from build123d import *

# Parameters (mm, degrees)
F0_R     = 9.95
F1_DEPTH = 3


with BuildPart() as f1:
    # F0 (on Top) → F1 (new body)
    with BuildSketch(Plane.XY):
        with BuildLine():
            ThreePointArc((14.825089, -2.284017), (14.743027, 2.764626), (12.990381, 7.5))
            ThreePointArc((12.990381, 7.5), (9.76575, 11.385523), (5.434528, 13.980912))
            ThreePointArc((5.434528, 13.980912), (0, 45.080944), (-5.434528, 13.980912))
            ThreePointArc((-5.434528, 13.980912), (-9.76575, 11.385523), (-12.990381, 7.5))
            ThreePointArc((-12.990381, 7.5), (-14.743027, 2.764626), (-14.825089, -2.284017))
            ThreePointArc((-14.825089, -2.284017), (-39.041242, -22.540472), (-9.390561, -11.696895))
            ThreePointArc((-9.390561, -11.696895), (-4.977277, -14.150149), (0, -15))
            ThreePointArc((0, -15), (4.977277, -14.150149), (9.390561, -11.696895))
            ThreePointArc((9.390561, -11.696895), (39.041242, -22.540472), (14.825089, -2.284017))
        make_face()
        with Locations((-25.163324, -14.528052)):
            Circle(F0_R, mode=Mode.SUBTRACT)
        with BuildLine():
            ThreePointArc((-9.526279, 5.5), (0, 11), (9.526279, 5.5))
            ThreePointArc((9.526279, 5.5), (9.526279, -5.5), (0, -11))
            ThreePointArc((0, -11), (-9.526279, -5.5), (-9.526279, 5.5))
        make_face(mode=Mode.SUBTRACT)
        with Locations((25.163324, -14.528052)):
            Circle(F0_R, mode=Mode.SUBTRACT)
        with Locations((0, 29.056104)):
            Circle(F0_R, mode=Mode.SUBTRACT)
    extrude(amount=F1_DEPTH)


solid = f1.part
Read the model definition and answer for the solid it produces. Units are mm, in the model's axes. Coordinates: 2 decimals unless noted, no trailing zeros. Loops run counter-clockwise (first coordinate to the right, second up) from the corner with the lowest first, then second, coordinate; pieces in that order, holes last. Notation, with made-up numbers: (-31.75, 82.25) -> (-27.75, 82.25) arc R31 cw to (-27.75, 109.25) -> close; hole circle Ø11 at (64.25, 48.25). An arc over 180 degrees is marked (long way). Answer in a Markdown table with one row per item.
Item 1: A cutting plane is placed at B-B on y = -6. Determine the outline of the cut face in (x, z), plus the area to 3 significant figures.
Returned:
| item | result |
|---|---|
| outline | (-38.73, 0) -> (-30.29, 0) -> (-30.29, 3) -> (-38.73, 3) -> close; (-20.04, 0) -> (-9.22, 0) -> (-9.22, 3) -> (-20.04, 3) -> close; (9.22, 0) -> (20.04, 0) -> (20.04, 3) -> (9.22, 3) -> close; (30.29, 0) -> (38.73, 0) -> (38.73, 3) -> (30.29, 3) -> close |
| area | 116 mm^2 |
Item 2: Each of these flat-tipped pins is pushed along its axis until it touches: P1, Ø16, axis at x = -25.16, y = -14.53, coming from the -Z side; P2, Ø1.5, axis at y = -20.5, z = 0.5, coming from the -X side. Where does it stop, or does it pass through?
Returned:
| item | result |
|---|---|
| P1 | passes through |
| P2 | stops at x = -40.31 |
Item 3: A cutting plane is placed at C-C on z = 1.1. Determine the outline of the cut face in (x, y), plus the area to 3 significant figures.
Returned:
| item | result |
|---|---|
| outline | (-14.83, -2.28) arc R16.02 ccw (long way) to (-9.39, -11.7) arc R15 ccw to (0, -15) arc R15 ccw to (9.39, -11.7) arc R16.02 ccw (long way) to (14.83, -2.28) arc R15 ccw to (12.99, 7.5) arc R15 ccw to (5.43, 13.98) arc R16.02 ccw (long way) to (-5.43, 13.98) arc R15 ccw to (-12.99, 7.5) arc R15 ccw to start; hole circle Ø19.9 at (-25.16, -14.53); hole circle Ø22 at (0, 0); hole circle Ø19.9 at (0, 29.06); hole circle Ø19.9 at (25.16, -14.53) |
| area | 1,770 mm^2 |
Item 4: A cutting plane is placed at A-A on x = -22. Determine the outline of the cut face in (y, z), plus the area to 3 significant figures.
Returned:
| item | result |
|---|---|
| outline | (-30.24, 0) -> (-23.96, 0) -> (-23.96, 3) -> (-30.24, 3) -> close; (-5.09, 0) -> (1.18, 0) -> (1.18, 3) -> (-5.09, 3) -> close |
| area | 37.7 mm^2 |
Item 5: A cutting plane is placed at D-D on y = 36.5. Determine the outline of the cut face in (x, z).
Returned:
| item | result |
|---|---|
| outline | (-14.19, 0) -> (-6.6, 0) -> (-6.6, 3) -> (-14.19, 3) -> close; (6.6, 0) -> (14.19, 0) -> (14.19, 3) -> (6.6, 3) -> close |
Item 6: For a pull along Y with two mould halves and no side action, classify faces 1 (the flat face through (9, -7, 3)), 2 (the cylindrical face through (34.654, -11.539, 1.479)), 3 (the cylindrical face through (0.63, 45.07, 1.48)) as released by +Y, released by -Y, zero draft, split by the parting line, or undercut.
Returned:
| item | result |
|---|---|
| face 1 | zero draft |
| face 2 | undercut |
| face 3 | undercut |
Item 7: Straight lines are drawn through the part: line 1 along X through (y, z) = (-10, 1.65); line 2 along X through (y, z) = (-20, 1.6); line 3 along Y through (x, z) = (9, 0.65). For each, find the intervals that lie inside material, in ascending order. Write a range as [from, to].
Returned:
| item | result |
|---|---|
| line 1 | x = [-40.54, -34.02], [-16.3, -4.58], [4.58, 16.3], [34.02, 40.54] |
| line 2 | x = [-40.22, -33.47], [-16.85, -10.1], [10.1, 16.85], [33.47, 40.22] |
| line 3 | y = [-12, -6.32], [6.32, 12], [15.8, 24.81], [33.3, 42.31] |
